Input: dimensioned drawing with shaded views. Units: mm. Origin: part minimum x, y, z. A direction names the side the tool comes from. Round coordinates to 2 decimals unless told otherwise and drop trailing zeros. Order: outer loops, then holes, each group sorted by start corner. A loop starts at its lowest first (then second) coordinate and runs counter-clockwise, first axis right, second up.
Item 1: Cut plane C-C on z = 5. Give the number of separate pieces and of enclosed holes in the cut face, then the cut area to 3 significant figures.
Item 2: First-contact query: pin 1 (5.5 mm diameter, centred on x = 57.15, y = 6.35, fed in from -Z) (3 decimals); pin 2 (3.5 mm diameter, centred on x = 69.85, y = 6.35, fed in from +Z); pin 3 (3 mm diameter, centred on x = 56.5, y = 1.5, fed in from +Z) (3 decimals); pin 4 (1 mm diameter, centred on y = 6.5, z = 1.5, fed in from +X). Flat tips, straight axial feed; report the tip coordinate or a pass-through.
Item 3: Line query: L1, parallel to X at y = 6.35, z = 7; L2, parallel to Y at x = 69.85, z = 5.5; L3, parallel to Z at x = 71, y = 4 (1 decimal). Output: solid intervals per line, ascending.
Item 4: Cut plane D-D on x = 6.35. Output: boundary loops of the cut face in (y, z).
Item 5: Cut plane A-A on x = 57.15. Output: boundary loops of the cut face in (y, z) (1 decimal).
Item 6: Cut plane B-B on y = 6.35. Output: boundary loops of the cut face in (x, z) (1 decimal).
Item 7: Reachability of the marked faces 1, 2 and 3 from +Z, -Z, +X, -X, +Y, -Y: full face, straight path, thin tool, end or side. Return the list, or none.
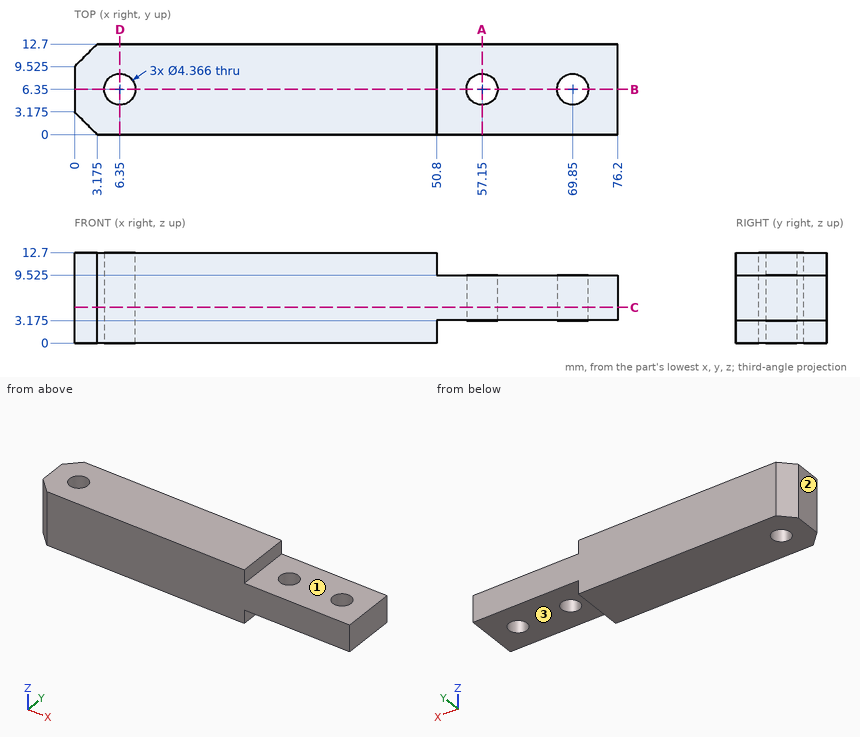
From the geometry:
1. separate pieces: 1
1. enclosed holes: 3
1. area: 913 mm2
2. pin 1: stops at z = 3.175
2. pin 2: passes through
2. pin 3: stops at z = 9.525
2. pin 4: stops at x = 50.8
3. L1: x = 0 to 4.17, 8.53 to 54.97, 59.33 to 67.67, 72.03 to 76.2
3. L2: y = 0 to 4.17, 8.53 to 12.7
3. L3: z = 3.2 to 9.5
4. outline: (0, 0) - (4.17, 0) - (4.17, 12.7) - (0, 12.7) - close; (8.53, 0) - (12.7, 0) - (12.7, 12.7) - (8.53, 12.7) - close
5. outline: (0, 3.2) - (4.2, 3.2) - (4.2, 9.5) - (0, 9.5) - close; (8.5, 3.2) - (12.7, 3.2) - (12.7, 9.5) - (8.5, 9.5) - close
6. outline: (0, 0) - (4.2, 0) - (4.2, 12.7) - (0, 12.7) - close; (8.5, 0) - (50.8, 0) - (50.8, 3.2) - (55, 3.2) - (55, 9.5) - (50.8, 9.5) - (50.8, 12.7) - (8.5, 12.7) - close; (59.3, 3.2) - (67.7, 3.2) - (67.7, 9.5) - (59.3, 9.5) - close; (72, 3.2) - (76.2, 3.2) - (76.2, 9.5) - (72, 9.5) - close
7. face 1: +Z, +X, +Y, -Y
7. face 2: +Z, -Z, -X, +Y, -Y
7. face 3: -Z, +X, +Y, -Y
